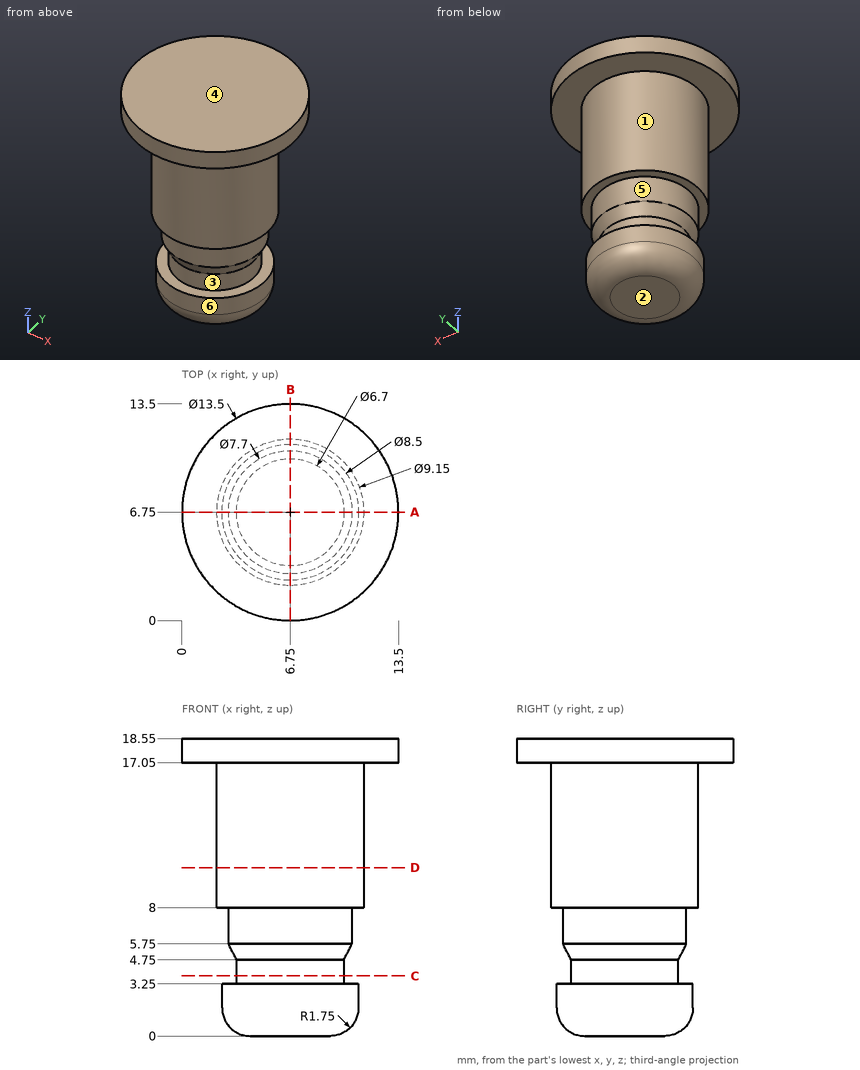
Geometry: see drawing. Coordinates: mm, zero at the bounding-box minimum. A direction names the side the tool comes from. Coordinates: 2 decimals unless noted, no trailing zeros. Write each loop counter-clockwise with the first axis right and the second up, starting at its lowest first coordinate (ties: lowest second). Pieces come first, ordered by that corner, then holes. Notation, with made-up numbers: (-30.75, 87.25) - (-22.75, 87.25) arc R11 ccw to (-22.75, 98.25) - close; hole circle Ø3 at (58, -6.75). An arc over 180 degrees is marked (long way). Put each result on its own line as item: value. Start each with the question number.
1) Ray query, L1, parallel to Z at x = 1.25, y = 10.5; L2, parallel to Z at x = 9.75, y = 4; L3, parallel to Y at x = 10.5, z = 2. Return the intervals inside material, ascending.
2) Cut plane D-D (z = 10.5). Return the cut outline in (x, y) (3 decimals), plus the area to 3 significant figures.
3) Contact query for flat-ended pins moving along their axis: pin 1 (4 mm diameter, centred on x = 4.5, y = 3, fed in from -Z); pin 2 (8 mm diameter, centred on y = 2.5, z = 14.5, fed in from -X); pin 3 (2 mm diameter, centred on x = 8, z = 8.5, fed in from +Y); pin 4 (5 mm diameter, centred on y = 9, z = 3, fed in from +X). Output: stop coordinate, or through.
4) Cut plane A-A (y = 6.75). Return the cut outline in (x, z) (3 decimals).
5) Mould query, pull axis Z, two halves, no side actions, for the marked faces 4, 5 and 6. Classes: pulls with the +Z half, pulls with the -Z half, needs draft (parallel to the pull), parting line crosses it, or undercut.
6) Cut plane C-C (z = 3.75). Return the cut outline in (x, y), plus the area to 3 significant figures.
7) Reachability of the marked faces 1, 2 and 3 from +Z, -Z, +X, -X, +Y, -Y: full face, straight path, thin tool, end or side. Return the list, or none.
Resolved:
1. L1: z = 17.05 to 18.55
1. L2: z = 0.98 to 3.25, 8 to 18.55
1. L3: y = 4.75 to 8.75
2. outline: circle Ø9.15 at (6.75, 6.75)
2. area: 65.8 mm2
3. pin 1: stops at z = 0
3. pin 2: stops at x = 0.1
3. pin 3: stops at y = 11.32
3. pin 4: stops at x = 11
4. outline: (0, 17.05) - (2.175, 17.05) - (2.175, 8) - (2.9, 8) - (2.9, 5.75) - (3.4, 4.75) - (3.4, 3.25) - (2.5, 3.25) - (2.5, 1.75) arc R1.75 ccw to (4.25, 0) - (9.25, 0) arc R1.75 ccw to (11, 1.75) - (11, 3.25) - (10.1, 3.25) - (10.1, 4.75) - (10.6, 5.75) - (10.6, 8) - (11.325, 8) - (11.325, 17.05) - (13.5, 17.05) - (13.5, 18.55) - (0, 18.55) - close
5. face 4: pulls with the +Z half
5. face 5: undercut
5. face 6: needs draft
6. outline: circle Ø6.7 at (6.75, 6.75)
6. area: 35.3 mm2
7. face 1: -Z
7. face 2: -Z, +X, -X, +Y, -Y
7. face 3: none
